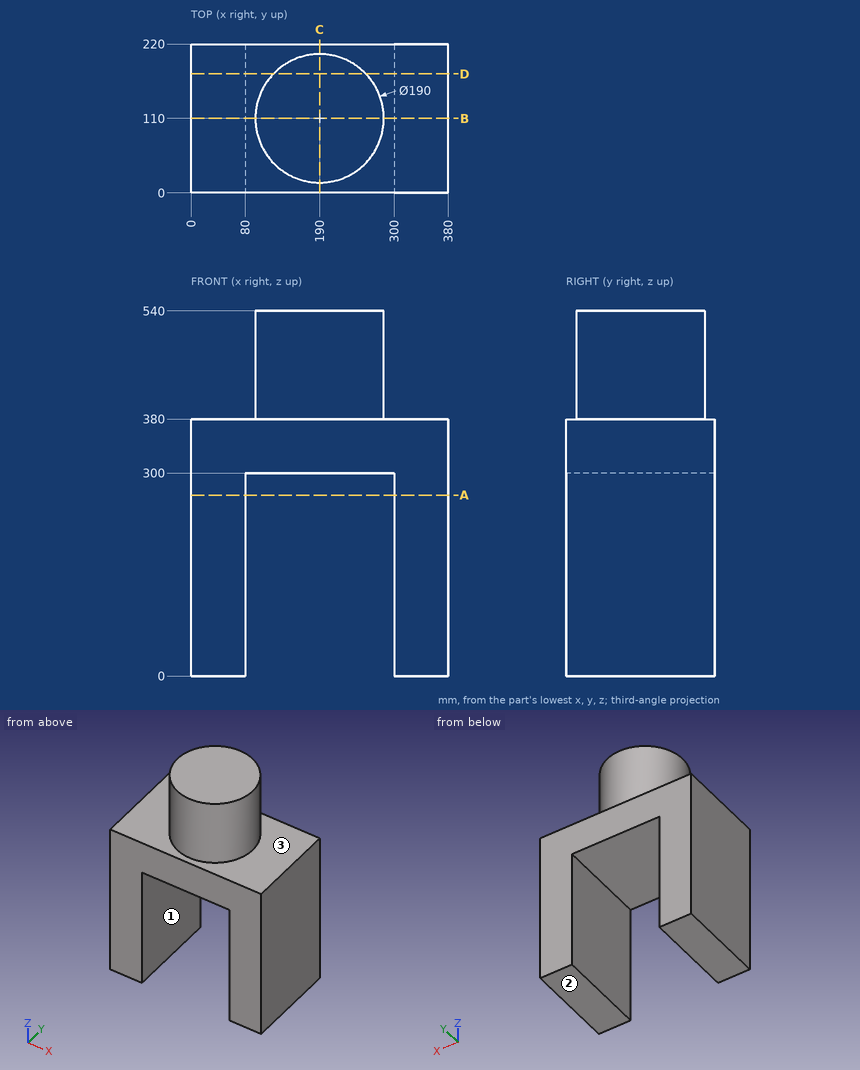
Design review of the part shown in the three views and the two pictorial views. Dimensions are in mm from the part's minimum x, y and z. A direction names the side the tool comes from. Coordinates: 2 decimals unless noted, no trailing zeros. Write each loop counter-clockwise with the first axis right and the second up, starting at its lowest first coordinate (ties: lowest second). Pieces come first, ordered by that corner, then holes.
(1) Wall thickness on probe 1 along X at (y, z) = (106, 36.5); probe 2 along Z at (x, y) = (175, 32.5); probe 3 along Z at (x, y) = (300.5, 100): over which ranges is each line inside the solid? List them lowest first.
(2) Add section D-D on y = 176. Give the boundary of the cut face in (x, z), then the cut area to 3 significant figures.
(3) Add section A-A on z = 267.5. Give the boundary of the cut face in (x, y), then the cut area to 3 significant figures.
(4) Add section B-B on y = 110. Give the boundary of the cut face in (x, z), then the cut area to 3 significant figures.
(5) For pin 1 Ø2 at (x, z) = (124, 340) entering from -Y; pin 2 Ø3 at (x, y) = (186.5, 30) entering from -Z, all flat-tipped, find the tip position at first contact; note any pin that passes through.
(6) Add section C-C on x = 190. Give the boundary of the cut face in (y, z).
(7) Tool access review of the marked faces 1, 2 and 3: name each direction out of +Z, -Z, +X, -X, +Y, -Y from which nothing blocks a thin tool from reaching the whole face with its end or side.
Answer sheet:
1. probe 1: x = 0 to 80, 300 to 380
1. probe 2: z = 300 to 540
1. probe 3: z = 0 to 380
2. outline: (0, 0) - (80, 0) - (80, 300) - (300, 300) - (300, 0) - (380, 0) - (380, 380) - (258.33, 380) - (258.33, 540) - (121.67, 540) - (121.67, 380) - (0, 380) - close
2. area: 100,000 mm2
3. outline: (0, 0) - (80, 0) - (80, 220) - (0, 220) - close; (300, 0) - (380, 0) - (380, 220) - (300, 220) - close
3. area: 35,200 mm2
4. outline: (0, 0) - (80, 0) - (80, 300) - (300, 300) - (300, 0) - (380, 0) - (380, 380) - (285, 380) - (285, 540) - (95, 540) - (95, 380) - (0, 380) - close
4. area: 109,000 mm2
5. pin 1: stops at y = 0
5. pin 2: stops at z = 300
6. outline: (0, 300) - (220, 300) - (220, 380) - (205, 380) - (205, 540) - (15, 540) - (15, 380) - (0, 380) - close
7. face 1: -Z, +Y, -Y
7. face 2: -Z, +X, -X, +Y, -Y
7. face 3: +Z
